Autodesk Inventor part; units mm, degrees
ref_plane "YZ Plane" through (0, 0, 0) normal (1, 0, 0) x (0, 1, 0)
ref_plane "XZ Plane" through (0, 0, 0) normal (0, 1, 0) x (-1, 0, 0)
ref_plane "XY Plane" through (0, 0, 0) normal (0, 0, 1) x (1, 0, 0)
sketch "Sketch1" plane through (0, 0, 0) normal (1, 0, 0) x (0, 1, 0)
  arc A0 (0, -277.0467) -> (138.5234, -239.9295) centre (0, 0) ccw
  arc A1 (0, -302.4467) -> (151.2234, -261.9266) centre (0, 0) ccw
  line L0 (138.5234, -239.9295) -> (151.2234, -261.9266)
  line L1 (0, -277.0467) -> (0, -302.4467)
  line L2 (127.3792, -246.0273) -> (140.2248, -268.2766)
  line L3 (140.2248, -268.2766) -> (162.2219, -255.5766)
  line L4 (162.2219, -255.5766) -> (149.5219, -233.5795)
  line L5 (149.5219, -233.5795) -> (127.5248, -246.2795)
  line L6 (127.5248, -246.2795) -> (162.2219, -255.5766) construction
  line L7 (140.2248, -268.2766) -> (149.5219, -233.5795) construction
  point P0 (144.8734, -250.928)
  point P1 (140.0915, -268.0455)
  dimension "d1" = 277.0467
  dimension "d2" = 30
  dimension "d4" = 25.4
  dimension "d5" = 25.4
extrude "Extrusion1" add sketch "Sketch1" along normal mid plane 177.8 contours A0 L2 A1 L1
sketch "Sketch2" plane through (-88.9, 0, -302.4467) normal (0, -1, 0) x (1, 0, 0)
  line L0 (177.8, 0) -> (0, 0)
  line L1 (177.8, 25.4) -> (177.8, 0)
  point P0 (88.9, 302.4467)
  point P1 (165.1, 12.7)
  dimension "d8" = 12.7
  dimension "d9" = 12.7
hole "Hole1" at (76.2, 0, -289.7467) direction (0, 1, 0) diameter 4.445 depth 38.1 counterbore diameter 5.588 counterbore depth 8.255
sketch "Sketch3" plane through (-88.9, 127.3792, -246.0273) normal (0, 0.866, 0.5) x (1, 0, 0)
  line L0 (88.9, 0) -> (88.9, 25.6912)
  line L1 (177.8, 25.4245) -> (177.8, 0)
  point P0 (88.9, -276.7555)
  point P1 (152.4, 12.9912)
  dimension "d17" = 25.4
  dimension "d18" = 12.7
hole "Hole2" at (63.5, 133.8748, -257.278) direction (0, -0.866, -0.5) diameter 4.445 depth 38.1 counterbore diameter 5.588 counterbore depth 8.255
pattern_linear "Rectangular Pattern1" count 7 spacing 25.4 along (-1, 0, 0) of "Hole1"
pattern_linear "Rectangular Pattern2" count 6 spacing 25.4 along (-1, 0, 0) of "Hole2"
properties part number "HoodBrace"
Work out the finished part from the listing and answer in its coordinate system (mm). A direction names the side the tool comes from. Coordinates: 2 decimals unless noted, no trailing zeros. Write each loop counter-clockwise with the first axis right and the second up, starting at its lowest first coordinate (ties: lowest second). Pieces come first, ordered by that corner, then holes.
Q1. Determine the mould class of faces 1 (the face through (-61.8, 131.36, -261.29)), 2 (the face through (-1.24, 66.45, -268.96)) for opening direction X: released by +X, released by -X, zero draft, split by the parting line, or undercut.
Q2. A cutting plane is placed at D-D, the plane y = 110. State how many separate pieces and enclosed holes the cut face has, then the cut area to 4 significant figures.
Q3. Which of the six approach directions +Z, -Z, +X, -X, +Y, -Y give full straight-line access (tool end or side, diameter ignored) to faces 3 (the face through (-1.2, 0, -286.7)), 4 (the face through (12.669, 100.864, -276.301)), 5 (the face through (-51, 38.1, -290))?
Q4. A cutting plane is placed at A-A, the plane y = 35.5. Give the vertices of the cut face in (x, z) (1 decimal), then the cut area to 3 significant figures.
Q5. A cutting plane is placed at B-B, the plane x = 76.2. Give the vertices of the cut face in (y, z) (3 decimals), then the cut area to 3 significant figures.
Q6. Each of these flat-tipped pins is pushed along its axis until it touches: pin 1 Ø1.3 at (x, z) = (-26, -290.5) entering from -Y; pin 2 Ø5 at (x, y) = (-3.5, 100.5) entering from +Z; pin 3 Ø1.5 at (x, z) = (-71, -255.5) entering from +Y. Where does it stop, or does it pass through?
Q7. Find the intervals of material crossed by line 1 (Z direction, x = 77.5, y = 31.5); line 2 (Z direction, x = 50.8, y = 5.5); line 3 (Z direction, x = 27, y = 77.5), in increasing order.
Q8. A cutting plane is placed at C-C, the plane y = 21. Give the vertices of the cut face in (x, z) (1 decimal).
Findings below:
1. face 1: undercut
1. face 2: zero draft
2. separate pieces: 1
2. enclosed holes: 6
2. area: 4,775 mm2
3. face 3: +Z, -Z, +X, -X, -Y
3. face 4: none
3. face 5: -Y
4. outline: (-88.9, -300.4) - (88.9, -300.4) - (88.9, -274.8) - (-88.9, -274.8) - close; hole circle Ø4.4 at (-76.2, -289.7); hole circle Ø4.4 at (-50.8, -289.7); hole circle Ø4.4 at (-25.4, -289.7); hole circle Ø4.4 at (0, -289.7); hole circle Ø4.4 at (25.4, -289.7); hole circle Ø4.4 at (50.8, -289.7); hole circle Ø4.4 at (76.2, -289.7)
4. area: 4,440 mm2
5. outline: (0, -302.447) arc R302.448 ccw to (140.091, -268.046) - (127.379, -246.027) arc R277.047 cw to (0, -277.047) - (0, -286.953) - (8.255, -286.953) - (8.255, -287.524) - (38.1, -287.524) - (38.1, -291.969) - (8.255, -291.969) - (8.255, -292.541) - (0, -292.541) - close
5. area: 3,350 mm2
6. pin 1: stops at y = 38.1
6. pin 2: stops at z = -257.19
6. pin 3: stops at y = 133.28
7. line 1: z = -300.8 to -291.55, -287.94 to -275.25
7. line 2: z = -302.4 to -292.54, -286.95 to -276.99
7. line 3: z = -292.35 to -265.99
8. outline: (-88.9, -301.7) - (88.9, -301.7) - (88.9, -276.2) - (-88.9, -276.2) - close; hole circle Ø4.4 at (-76.2, -289.7); hole circle Ø4.4 at (-50.8, -289.7); hole circle Ø4.4 at (-25.4, -289.7); hole circle Ø4.4 at (0, -289.7); hole circle Ø4.4 at (25.4, -289.7); hole circle Ø4.4 at (50.8, -289.7); hole circle Ø4.4 at (76.2, -289.7)
